Can you work these out from the model? Positions are in its coordinate system, mm. A direction names the side the tool comes from. Give positions to 0.01 mm unless a question says otherwise; leave off trailing zeros. Loops run counter-clockwise (first coordinate to the right, second up) from the corner with the lowest first, then second, coordinate; pieces in that order, holes last. Notation, with made-up numbers: (6.5, 63.25) -> (20.5, 63.25) arc R14 ccw to (20.5, 88.25) -> close; hole circle Ø8 at (89.25, 34.5). An arc over 180 degrees is marked (long way). One line per question, with ' | ' between items.
from build123d import *

# Parameters (mm, degrees)
F0_R     = 2.5
F1_DEPTH = 7.5
F2_R     = 2.5
F4_DEPTH = 1
F5_W     = 0.5
F5_H     = 0.5
F6_DEPTH = 5.5


with BuildPart() as f1:
    # F0 (on Top) → F1 (new body)
    with BuildSketch(Plane.XY):
        Circle(F0_R)
    extrude(amount=F1_DEPTH)

    # F2
    f2_edges = [f1.edges().sort_by_distance(p)[0] for p in [
        (-2.5, 0, 7.5),
    ]]
    fillet(f2_edges, radius=F2_R)

    # F3 (on face) → F4 (join)
    with BuildSketch(Plane(origin=(0, 0, 0), x_dir=(1, 0, 0), z_dir=(0, 0, -1))):
        with BuildLine():
            Line((-1.260952, -2.5), (1.260952, -2.5))
            ThreePointArc((1.260952, -2.5), (0, 2.8), (-1.260952, -2.5))
        make_face()
    extrude(amount=F4_DEPTH)

    # F5 (on face) → F6 (join)
    with BuildSketch(Plane(origin=(0, 0, -1), x_dir=(1, 0, 0), z_dir=(0, 0, -1))):
        Rectangle(F5_W, F5_H)
    extrude(amount=F6_DEPTH)

    # F8: sweep along a path in F7
    with BuildLine(Plane.YZ) as f8_path:
        Line((-1.75, -1), (-1.75, -1.326328))
        ThreePointArc((-1.75, -1.326328), (-1.777681, -1.490385), (-1.857659, -1.636277))
        Line((-1.857659, -1.636277), (-2.432341, -2.363723))
        ThreePointArc((-2.432341, -2.363723), (-2.512319, -2.509615), (-2.54, -2.673672))
        Line((-2.54, -2.673672), (-2.54, -6.5))
    # F5 (on face) → F8 (sweep)
    with BuildSketch(Plane(origin=(0, 0, -1), x_dir=(1, 0, 0), z_dir=(0, 0, -1))):
        with Locations((0, 1.75)):
            Rectangle(F5_W, F5_H)
    sweep(path=f8_path.line)

    # F9: sweep along a path in F7
    with BuildLine(Plane.YZ) as f9_path:
        Line((1.75, -1), (1.75, -1.326328))
        ThreePointArc((1.75, -1.326328), (1.777681, -1.490385), (1.857659, -1.636277))
        Line((1.857659, -1.636277), (2.432341, -2.363723))
        ThreePointArc((2.432341, -2.363723), (2.512319, -2.509615), (2.54, -2.673672))
        Line((2.54, -2.673672), (2.54, -6.5))
    # F5 (on face) → F9 (sweep)
    with BuildSketch(Plane(origin=(0, 0, -1), x_dir=(1, 0, 0), z_dir=(0, 0, -1))):
        with Locations((0, -1.75)):
            Rectangle(F5_W, F5_H)
    sweep(path=f9_path.line)


solid = f1.part
Q1. If we section it at D-D (z = 1.5): Write out the boundary of the cut face in (x, y).
Entries:
outline: circle Ø5 at (0, 0)
Q2. If we section it at A-A (z = -4.75): Write out the boundary of the cut face in (x, y), plus the area to 3 significant figures.
Entries:
outline: (-0.25, -2.79) -> (0.25, -2.79) -> (0.25, -2.29) -> (-0.25, -2.29) -> close; (-0.25, -0.25) -> (0.25, -0.25) -> (0.25, 0.25) -> (-0.25, 0.25) -> close; (-0.25, 2.29) -> (0.25, 2.29) -> (0.25, 2.79) -> (-0.25, 2.79) -> close | area: 0.750 mm²
Q3. If I drill on probe 1 along X at (y, z) = (-0.2, -1.75); probe 2 along Y at (x, z) = (-2.3, 1); probe 3 along Z at (x, y) = (1.2, -0.7), over which ranges is the centre line in solid material (lowest first)? Write a range as from..to.
Entries:
probe 1: -0.25..0.25 | probe 2: -0.98..0.98 | probe 3: -1..7.08
Q4. For pin 1 Ø1 at (x, z) = (-1, 1.5) entering from -Y; pin 2 Ø1.4 at (y, z) = (2.5, -4.5) entering from +X; pin 3 Ø1.4 at (y, z) = (-2, -4) entering from -X, each with a flat end and sliding along its axis, tell me the tip position at first contact or that it passes through.
Entries:
pin 1: y = -2.45 | pin 2: x = 0.25 | pin 3: x = -0.25
Q5. On a 3-axis mill with a long thin cutter (end or side, diameter ignored), from which of +Z, -Z, +X, -X, +Y, -Y can I reach the whole of each face in a straight line? I mean faces 1 (the face through (-0.54, -2.44, 2.46)), 2 (the face through (-0.25, -2.441, -3.788)), 3 (the face through (0.1, -2.8, -0.5)), 4 (the face through (0.25, 2.441, -3.788)). Say none if no direction works.
Entries:
face 1: +Z | face 2: -Z, -X, +Y, -Y | face 3: +Z, -Z | face 4: -Z, +X, +Y, -Y
Q6. If we section it at B-B (y = 0): Write out the boundary of the cut face in (x, z), plus the area to 3 significant figures.
Entries:
outline: (-2.8, -1) -> (-0.25, -1) -> (-0.25, -6.5) -> (0.25, -6.5) -> (0.25, -1) -> (2.8, -1) -> (2.8, 0) -> (2.5, 0) -> (2.5, 5) arc R2.5 ccw to (-2.5, 5) -> (-2.5, 0) -> (-2.8, 0) -> close | area: 43.2 mm²
Q7. If we section it at C-C (x = -2.25): Write out the boundary of the cut face in (y, z), plus the area to 3 significant figures.
Entries:
outline: (-1.67, -1) -> (1.67, -1) -> (1.67, 0) -> (1.09, 0) -> (1.09, 5) arc R1.09 ccw to (-1.09, 5) -> (-1.09, 0) -> (-1.67, 0) -> close | area: 16.1 mm²
